Autodesk Inventor part; units mm, degrees
ref_plane "YZ Plane" through (0, 0, 0) normal (1, 0, 0) x (0, 1, 0)
ref_plane "XZ Plane" through (0, 0, 0) normal (0, 1, 0) x (-1, 0, 0)
ref_plane "XY Plane" through (0, 0, 0) normal (0, 0, 1) x (1, 0, 0)
sketch "Sketch1" plane through (0, 0, 0) normal (0, 0, 1) x (1, 0, 0)
  circle A0 centre (0, 0) radius 5.5
  dimension "d0" = 11
extrude "Extrusion1" add sketch "Sketch1" along normal blind 5
sketch "Sketch2" plane through (0, 0, 5) normal (0, 0, 1) x (1, 0, 0)
  circle A0 centre (0, 0) radius 5.5
  line L0 (0, 0) -> (-1, 0)
  circle A1 centre (-1, 0) radius 1.75
  circle A2 centre (-1, 0) radius 3.4167
  dimension "d5" = 1
  dimension "d6" = 3.5
  dimension "d7" = 1.6667
extrude "Extrusion2" add sketch "Sketch2" along normal blind 1 contours A2
sketch "Sketch3" plane through (-1, 0, 5) normal (0, 0, 1) x (1, 0, 0)
  circle A0 centre (0, 0) radius 1.75
  point P0 (1, 0)
extrude "Extrusion3" cut sketch "Sketch3" against normal through all
properties part number "eccentric stop"
The listing builds one solid part. Answer for the finished solid, in the listing's coordinates (mm). A direction names the side the tool comes from. Give positions to 0.01 mm unless a question says otherwise; leave off trailing zeros. Loops run counter-clockwise (first coordinate to the right, second up) from the corner with the lowest first, then second, coordinate; pieces in that order, holes last. Notation, with made-up numbers: (10.25, 30.5) - (40.25, 30.5) arc R15 cw to (40.25, 55.5) - close; hole circle Ø4 at (71, 42.5). An arc over 180 degrees is marked (long way). Use one line per item in the form item = value.
1. Section C-C on z = 3.25 is taken. Give the vertices of the cut face in (x, y), then the cut area to 3 significant figures.
Calculated:
outline = circle Ø11 at (0, 0); hole circle Ø3.5 at (-1, 0)
area = 85.4 mm^2
2. Section A-A on y = 0 is taken. Give the vertices of the cut face in (x, z), then the cut area to 3 significant figures.
Calculated:
outline = (-5.5, 0) - (-2.75, 0) - (-2.75, 6) - (-4.42, 6) - (-4.42, 5) - (-5.5, 5) - close; (0.75, 0) - (5.5, 0) - (5.5, 5) - (2.42, 5) - (2.42, 6) - (0.75, 6) - close
area = 40.8 mm^2
3. Which of the six approach directions +Z, -Z, +X, -X, +Y, -Y give full straight-line access (tool end or side, diameter ignored) to faces 1 (the face through (0.58, 3.03, 5.49)), 2 (the face through (-1.19, 5.37, 2.46))?
Calculated:
face_1 = +Z
face_2 = +Z, -Z
4. Find the intervals of material crossed by line 1 along X through (y, z) = (0.75, 0.6); line 2 along Z through (x, y) = (-3.5, 2.75); line 3 along Y through (x, z) = (0.5, 2.3), in increasing order. Write a range as [from, to].
Calculated:
line_1 = [-5.45, -2.58], [0.58, 5.45]
line_2 = [0, 5]
line_3 = [-5.48, -0.9], [0.9, 5.48]
5. Section B-B on x = 0.5 is taken. Give the vertices of the cut face in (y, z).
Calculated:
outline = (-5.48, 0) - (-0.9, 0) - (-0.9, 6) - (-3.07, 6) - (-3.07, 5) - (-5.48, 5) - close; (0.9, 0) - (5.48, 0) - (5.48, 5) - (3.07, 5) - (3.07, 6) - (0.9, 6) - close
6. Section D-D on y = -3.25 is taken. Give the vertices of the cut face in (x, z).
Calculated:
outline = (-4.44, 0) - (4.44, 0) - (4.44, 5) - (0.05, 5) - (0.05, 6) - (-2.05, 6) - (-2.05, 5) - (-4.44, 5) - close
